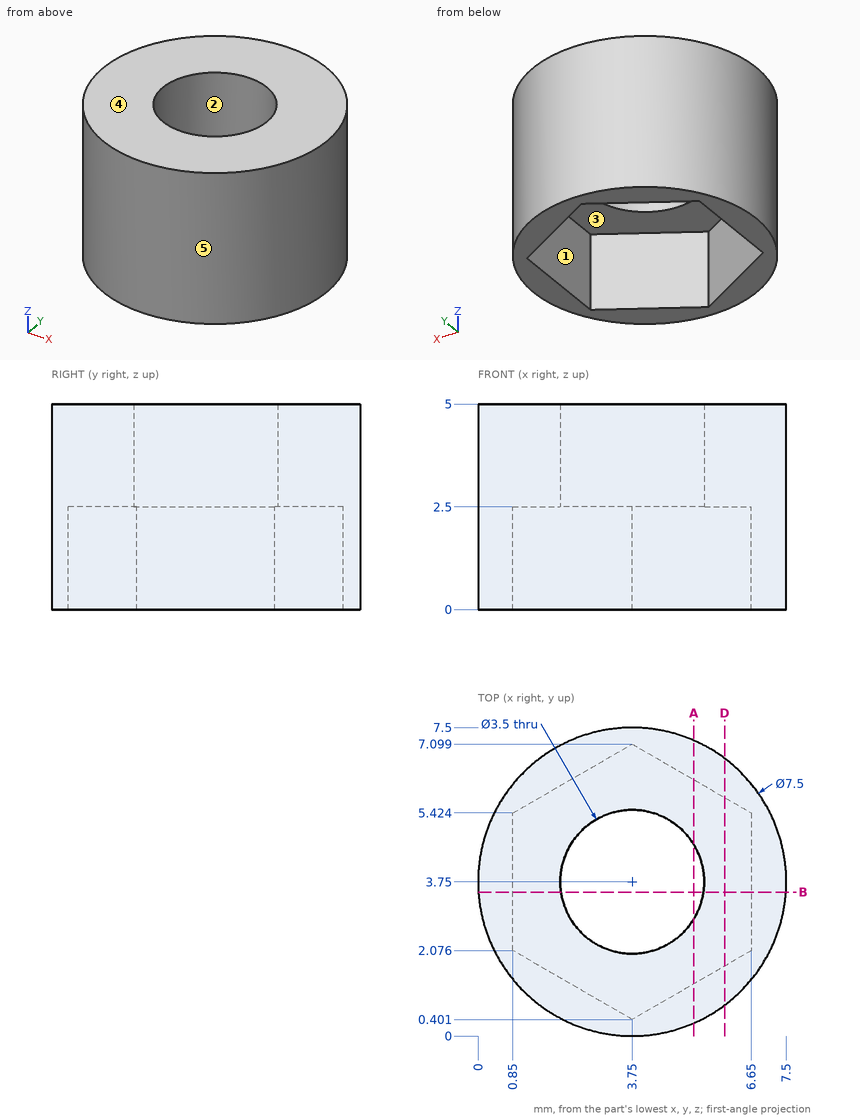
Could you check a few things on this drawing? It's one solid part, dimensions in mm from its lowest x, y, z. A direction names the side the tool comes from. Round coordinates to 2 decimals unless told otherwise and drop trailing zeros. Loops run counter-clockwise (first coordinate to the right, second up) from the corner with the lowest first, then second, coordinate; pieces in that order, holes last. Notation, with made-up numbers: M -21,67.25 L -12,67.25 A18 cw -12,84.25 Z; hole C 17,-24 d4. An arc over 180 degrees is marked long. Write item = value, one per line. Start each with the question number.
(1) I'm going to push flat-ended pins straight in: P1, Ø3, axis at y = 3, z = 1.5, coming from the +X side; P2, Ø1.5, axis at y = 1, z = 4, coming from the -X side; P3, Ø1, axis at y = 6.5, z = 2, coming from the -X side; P4, Ø3, axis at x = 3.75, y = 3.75, coming from the -Z side. Where does each tip first touch, or does it pass through?
(2) I need wall thicknesses on line 1 along Y through (x, z) = (3.75, 3.5); line 2 along Z through (x, y) = (4.25, 1.25); line 3 along X through (y, z) = (7, 1.35). Which ranges of each line are inside material? Lowest first, please.
(3) If we mould it in two halves opening along X, with no side actions, what happens to the marked faces 3, 4 and 5? For each: released by +X, released by -X, zero draft, split by the parting line, or undercut.
(4) Suppose I cut it at A-A on x = 5.25. Write out the boundary of the cut face in (y, z).
(5) Suppose I cut it at B-B on y = 3.5. Write out the boundary of the cut face in (x, z).
(6) Suppose I cut it at D-D on x = 6. Write out the boundary of the cut face in (y, z).
(7) Which directions (+Z, -Z, +X, -X, +Y, -Y) give clear straight access to the entire face, cutting with the end or side of a thin tool? Please do the marked faces 1 and 2.
Answer block:
q1.P1 = 7.5
q1.P2 = 0.58
q1.P3 = 0.75
q1.P4 = through
q2.line_1 = 0 to 2, 5.5 to 7.5
q2.line_2 = 2.5 to 5
q2.line_3 = 1.88 to 3.58, 3.92 to 5.62
q3.face_3 = undercut
q3.face_4 = zero draft
q3.face_5 = split by the parting line
q4.outline = M 0.31,0 L 1.27,0 L 1.27,2.5 L 2.85,2.5 L 2.85,5 L 0.31,5 Z; M 4.65,2.5 L 6.23,2.5 L 6.23,0 L 7.19,0 L 7.19,5 L 4.65,5 Z
q5.outline = M 0.01,0 L 0.85,0 L 0.85,2.5 L 2.02,2.5 L 2.02,5 L 0.01,5 Z; M 5.48,2.5 L 6.65,2.5 L 6.65,0 L 7.49,0 L 7.49,5 L 5.48,5 Z
q6.outline = M 0.75,0 L 1.7,0 L 1.7,2.5 L 5.8,2.5 L 5.8,0 L 6.75,0 L 6.75,5 L 0.75,5 Z
q7.face_1 = -Z
q7.face_2 = +Z, -Z
